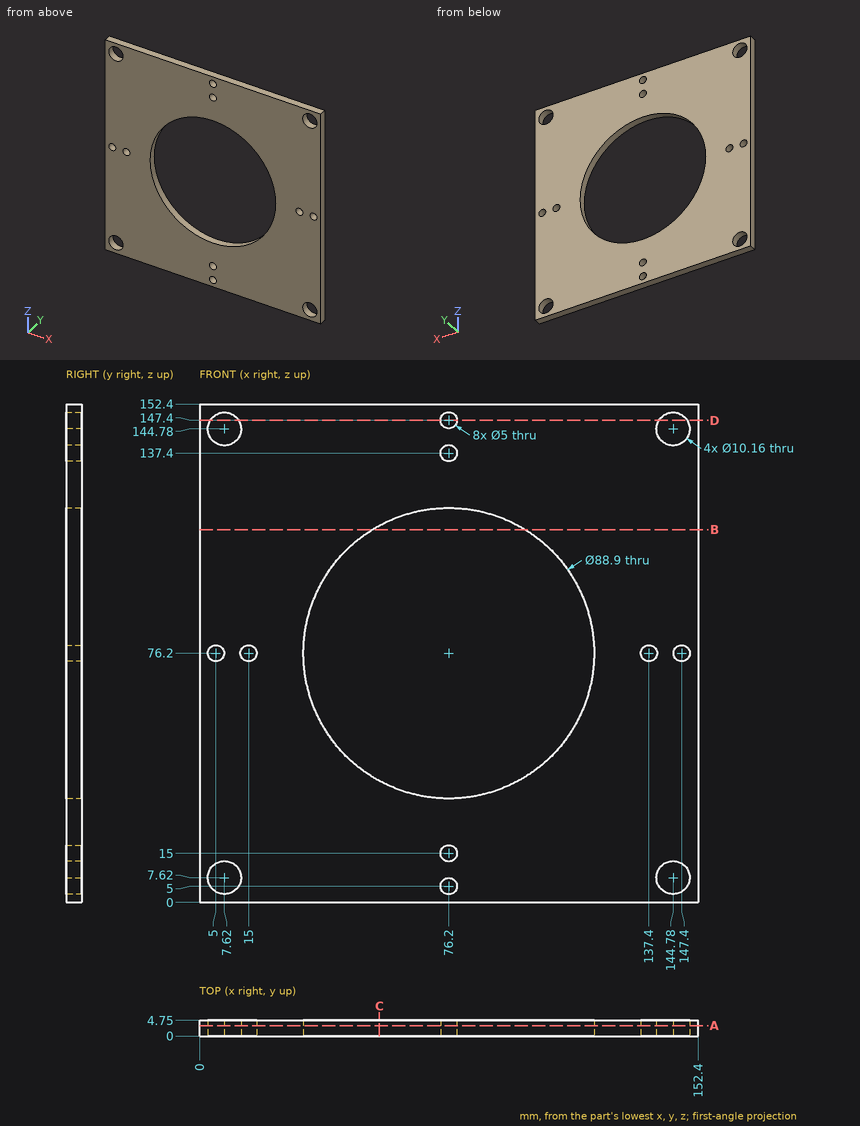
Verification items for this drawing (mm, ordinates from the low corner). Coordinates: 2 decimals unless noted, no trailing zeros. Order: outer loops, then holes, each group sorted by start corner. A loop starts at its lowest first (then second) coordinate and runs counter-clockwise, first axis right, second up. Notation, with made-up numbers: M 58,47 L 97,47 A18 cw 97,76 Z; hole C 63,48.25 d4. An arc over 180 degrees is marked long. Answer as a JSON object with one key per item and string values.
Q1. Cross-section at A-A on y = 3.2. Give the number of separate pieces and of enclosed holes in the cut face, and give its area (3 significant figures).
Results are:
{"separate pieces": "1", "enclosed holes": "13", "area": "16,500 mm²"}
Q2. Scan lines: line 1 (X direction, y = 3.1, z = 7.62); line 2 (X direction, y = 3.4, z = 76.2); line 3 (Z direction, x = 146, y = 4). Record each from-to range of solid material in increasing order.
Results are:
{"line 1": "x = 0 to 2.54, 12.7 to 139.7, 149.86 to 152.4", "line 2": "x = 0 to 2.5, 7.5 to 12.5, 17.5 to 31.75, 120.65 to 134.9, 139.9 to 144.9, 149.9 to 152.4", "line 3": "z = 0 to 2.69, 12.55 to 74.13, 78.27 to 139.85, 149.71 to 152.4"}
Q3. Depth check by flat-ended pin: pin 1 Ø4 at (x, z) = (5, 76.2) entering from +Y. Enter the tip coordinate at first touch or a pass-through.
Results are:
{"pin 1": "passes through"}
Q4. Cross-section at B-B on z = 114. Record the cut outline in (x, y).
Results are:
{"outline": "M 0,0 L 52.81,0 L 52.81,4.75 L 0,4.75 Z; M 99.59,0 L 152.4,0 L 152.4,4.75 L 99.59,4.75 Z"}
Q5. Cross-section at D-D on z = 147.4. Record the cut outline in (x, y).
Results are:
{"outline": "M 0,0 L 3.27,0 L 3.27,4.75 L 0,4.75 Z; M 11.97,0 L 73.7,0 L 73.7,4.75 L 11.97,4.75 Z; M 78.7,0 L 140.43,0 L 140.43,4.75 L 78.7,4.75 Z; M 149.13,0 L 152.4,0 L 152.4,4.75 L 149.13,4.75 Z"}
Q6. Cross-section at C-C on x = 55. Record the cut outline in (y, z).
Results are:
{"outline": "M 0,0 L 4.75,0 L 4.75,37.13 L 0,37.13 Z; M 0,115.27 L 4.75,115.27 L 4.75,152.4 L 0,152.4 Z"}
